Part model, mm, in its own coordinate system. A direction names the side the tool comes from. Give positions to 0.01 mm unless a question says otherwise; leave off trailing zeros. Order: outer loops, then holes, each group sorted by start corner. A loop starts at its lowest first (then second) coordinate and runs counter-clockwise, first axis right, second up. Notation, with made-up numbers: (-27.5, 77.25) - (14.5, 77.25) arc R34 cw to (14.5, 112.25) - close; hole circle Ø1 at (84.25, 36). An arc over 180 degrees is marked (long way). Use a Markdown table: item, result. Add a question column.
Autodesk Inventor part; units mm, degrees
ref_plane "YZ Plane" through (0, 0, 0) normal (1, 0, 0) x (0, 1, 0)
ref_plane "XZ Plane" through (0, 0, 0) normal (0, 1, 0) x (-1, 0, 0)
ref_plane "XY Plane" through (0, 0, 0) normal (0, 0, 1) x (1, 0, 0)
sketch "Sketch1" plane through (0, 0, 0) normal (0, 0, 1) x (1, 0, 0)
  line L0 (0, 70) -> (0, -70) construction
  line L1 (-153.5, 0) -> (91.5, 0) construction
  line L2 (-118.5, 50) -> (56.5, 50)
  line L3 (56.5, 50) -> (56.5, -50)
  line L4 (56.5, -50) -> (-118.5, -50)
  line L5 (-118.5, -50) -> (-118.5, 50)
  point P0 (0, 0)
  dimension "d0" = 100
  dimension "d1" = 56.5
  dimension "d2" = 175
extrude "Extrusion1" add sketch "Sketch1" along normal blind 12.5
sketch "Sketch2" plane through (0, 0, 12.5) normal (0, 0, 1) x (1, 0, 0)
  line L0 (56.5, 50) -> (-118.5, 50) construction
  line L1 (-118.5, 50) -> (-118.5, -50) construction
  line L2 (-118.5, -50) -> (56.5, -50) construction
  line L3 (56.5, -50) -> (56.5, 50) construction
  line L4 (0, 70) -> (0, -70) construction
  line L5 (-153.5, 0) -> (91.5, 0) construction
  line L6 (-37.5, 37.5) -> (37.5, 37.5) construction
  line L7 (37.5, 37.5) -> (37.5, -37.5) construction
  line L8 (37.5, -37.5) -> (-37.5, -37.5) construction
  line L9 (-37.5, -37.5) -> (-37.5, 37.5) construction
  point P0 (0, 0)
  dimension "d5" = 75
  dimension "d6" = 75
hole "Hole1" at (-37.5, 37.5, 12.5) at (-37.5, -37.5, 12.5) at (37.5, -37.5, 12.5) at (37.5, 37.5, 12.5) direction (0, 0, -1) diameter 6 end through all counterbore diameter 10.5 counterbore depth 7
sketch "Sketch3" plane through (0, 0, 12.5) normal (0, 0, 1) x (1, 0, 0)
  circle A0 centre (-37.5, -37.5) radius 5.25 construction
  circle A1 centre (-37.5, 37.5) radius 5.25 construction
  circle A2 centre (37.5, -37.5) radius 5.25 construction
  line L0 (56.5, 50) -> (-118.5, 50) construction
  line L1 (-118.5, 50) -> (-118.5, -50) construction
  line L2 (-118.5, -50) -> (56.5, -50) construction
  line L3 (56.5, -50) -> (56.5, 50) construction
  line L4 (-153.5, 0) -> (91.5, 0) construction
  line L5 (0, 70) -> (0, -70) construction
  point P0 (0, 0)
  point P1 (25, 25)
  point P2 (0, 25)
  point P3 (-25, 25)
  point P4 (-50, 25)
  point P5 (-75, 25)
  point P6 (-100, 25)
  point P7 (25, 0)
  point P8 (0, 0)
  point P9 (-25, 0)
  point P10 (-50, 0)
  point P11 (-75, 0)
  point P12 (-100, 0)
  point P13 (25, -25)
  point P14 (0, -25)
  point P15 (-25, -25)
  point P16 (-50, -25)
  point P17 (-75, -25)
  point P18 (-100, -25)
  dimension "d14" = 25
  dimension "d15" = 25
  dimension "d18" = 25
  dimension "d21" = 25
hole "Hole2" at (0, 0, 12.5) at (25, 25, 12.5) at (0, 25, 12.5) at (-25, 25, 12.5) at (-50, 25, 12.5) at (-75, 25, 12.5) at (-100, 25, 12.5) at (25, 0, 12.5) at (-25, 0, 12.5) at (-50, 0, 12.5) at (-75, 0, 12.5) at (-100, 0, 12.5) at (25, -25, 12.5) at (0, -25, 12.5) at (-25, -25, 12.5) at (-50, -25, 12.5) at (-75, -25, 12.5) at (-100, -25, 12.5) direction (0, 0, -1) diameter 4.917 end through all
properties part number "M605-to-X95-adapter-V1"
1. Cut at D-D (y = -25). Write the cut outline in (x, z), plus the area to 3 significant figures.
2. Pin check, flat tips, straight feed: P1, Ø9.5, axis at x = 37.5, y = 37.5, coming from the +Z side; P2, Ø8, axis at x = -25, y = 25, coming from the +Z side. Stop position of each tip, or through.
3. Cut at C-C (x = 25). Write the cut outline in (y, z).
4. Drill centre lines: probe 1 along X at (y, z) = (-37.5, 8.25); probe 2 along Y at (x, z) = (0, 9.75); probe 3 along X at (y, z) = (-33, 7.5). Where is each one in solid material? Low to high. Write a range as [from, to].
5. Tool access for faces 4 (the face through (-97.6, 0.53, 6.16)), 5 (the face through (-41.05, 41.37, 8.95)): list every direction of +Z, -Z, +X, -X, +Y, -Y with a clear straight run to the whole face (end or side of a thin tool).
6. Cut at B-B (z = 2). State how many separate pieces and enclosed holes the cut face has, plus the area to 3 significant figures.
7. Mould opens along Y. For faces 1 (the face through (-97.6, 25.53, 6.16)), 2 (the face through (-118.5, -1, 6)), 3 (the face through (40, -40, 5.5)) say: released by +Y, released by -Y, zero draft, split by the parting line, or undercut.
8. Cut at A-A (y = 37.5). Write the cut outline in (x, z).
Responses:
| question | item | result |
|---|---|---|
| 1 | outline | (-118.5, 0) - (-102.46, 0) - (-102.46, 12.5) - (-118.5, 12.5) - close; (-97.54, 0) - (-77.46, 0) - (-77.46, 12.5) - (-97.54, 12.5) - close; (-72.54, 0) - (-52.46, 0) - (-52.46, 12.5) - (-72.54, 12.5) - close; (-47.54, 0) - (-27.46, 0) - (-27.46, 12.5) - (-47.54, 12.5) - close; (-22.54, 0) - (-2.46, 0) - (-2.46, 12.5) - (-22.54, 12.5) - close; (2.46, 0) - (22.54, 0) - (22.54, 12.5) - (2.46, 12.5) - close; (27.46, 0) - (56.5, 0) - (56.5, 12.5) - (27.46, 12.5) - close |
| 1 | area | 1,820 mm² |
| 2 | P1 | stops at z = 5.5 |
| 2 | P2 | stops at z = 12.5 |
| 3 | outline | (-50, 0) - (-27.46, 0) - (-27.46, 12.5) - (-50, 12.5) - close; (-22.54, 0) - (-2.46, 0) - (-2.46, 12.5) - (-22.54, 12.5) - close; (2.46, 0) - (22.54, 0) - (22.54, 12.5) - (2.46, 12.5) - close; (27.46, 0) - (50, 0) - (50, 12.5) - (27.46, 12.5) - close |
| 4 | probe 1 | x = [-118.5, -42.75], [-32.25, 32.25], [42.75, 56.5] |
| 4 | probe 2 | y = [-50, -27.46], [-22.54, -2.46], [2.46, 22.54], [27.46, 50] |
| 4 | probe 3 | x = [-118.5, -40.2], [-34.8, 34.8], [40.2, 56.5] |
| 5 | face 4 | +Z, -Z |
| 5 | face 5 | +Z |
| 6 | separate pieces | 1 |
| 6 | enclosed holes | 22 |
| 6 | area | 17,000 mm² |
| 7 | face 1 | undercut |
| 7 | face 2 | zero draft |
| 7 | face 3 | undercut |
| 8 | outline | (-118.5, 0) - (-40.5, 0) - (-40.5, 5.5) - (-42.75, 5.5) - (-42.75, 12.5) - (-118.5, 12.5) - close; (-34.5, 0) - (34.5, 0) - (34.5, 5.5) - (32.25, 5.5) - (32.25, 12.5) - (-32.25, 12.5) - (-32.25, 5.5) - (-34.5, 5.5) - close; (40.5, 0) - (56.5, 0) - (56.5, 12.5) - (42.75, 12.5) - (42.75, 5.5) - (40.5, 5.5) - close |
